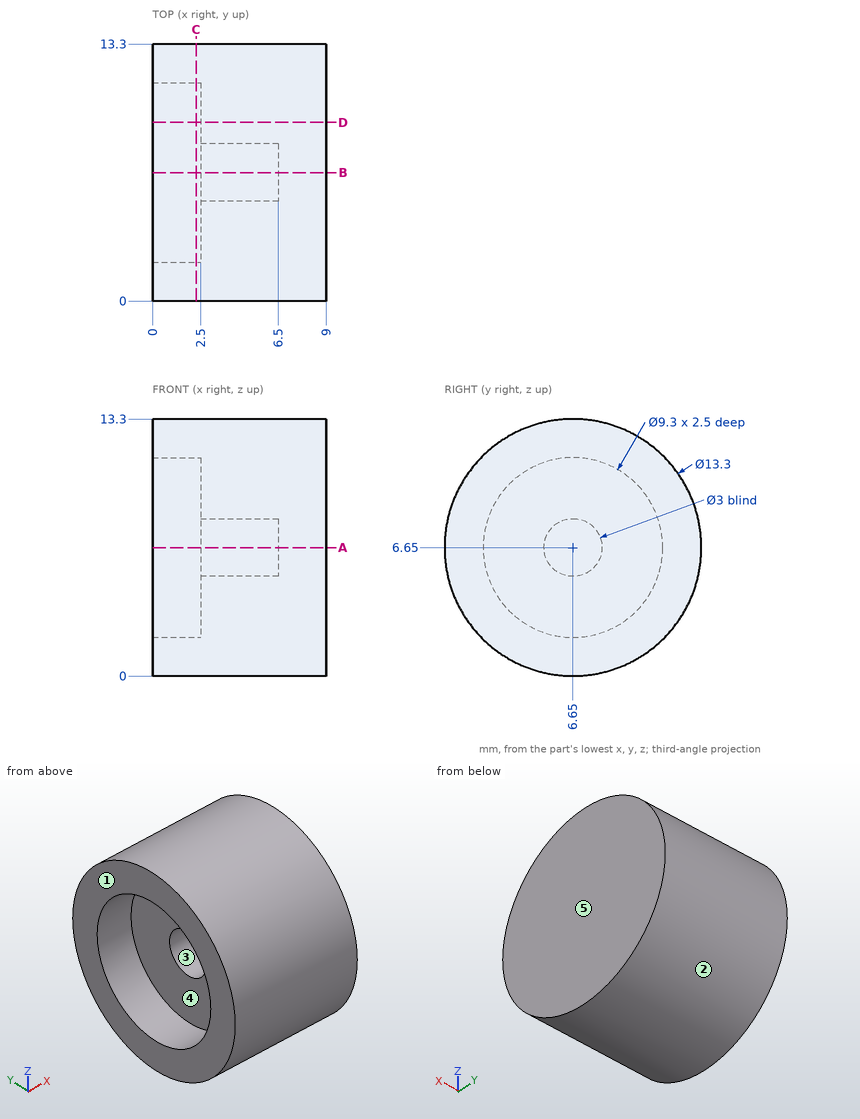
Geometry: see drawing. Coordinates: mm, zero at the bounding-box minimum. A direction names the side the tool comes from. Round coordinates to 2 decimals unless told otherwise and drop trailing zeros. Write each loop counter-clockwise with the first axis right and the second up, starting at its lowest first coordinate (ties: lowest second). Pieces come first, ordered by that corner, then holes.
1) Reachability of the marked faces 4 and 5 from +Z, -Z, +X, -X, +Y, -Y: full face, straight path, thin tool, end or side. Return the list, or none.
2) Draft query along Y for the marked faces 1, 2 and 3. Return one class per face: pulls with the +Y half, pulls with the -Y half, needs draft (parallel to the pull), parting line crosses it, or undercut.
3) Cut plane A-A (z = 6.65). Return the cut outline in (x, y).
4) Contact query for flat-ended pins moving along their axis: P1, Ø1, axis at x = 5.5, z = 9, coming from the -Y side; P2, Ø1.5, axis at y = 7, z = 7, coming from the -X side; P3, Ø2, axis at x = 2.5, y = 9, coming from the -Z side. Output: stop coordinate, or through.
5) Ray query, L1, parallel to Z at x = 1.35, y = 6.65; L2, parallel to X at y = 6, z = 4.5; L3, parallel to Z at x = 2, y = 2.75. Return the intervals inside material, ascending.
6) Cut plane C-C (x = 2.25). Return the cut outline in (y, z), then the cut area to 3 significant figures.
7) Cut plane D-D (y = 9.25). Return the cut outline in (x, z).
Geometry says:
1. face 4: -X
1. face 5: +Z, -Z, +X, +Y, -Y
2. face 1: needs draft
2. face 2: parting line crosses it
2. face 3: undercut
3. outline: (0, 0) - (9, 0) - (9, 13.3) - (0, 13.3) - (0, 11.3) - (2.5, 11.3) - (2.5, 8.15) - (6.5, 8.15) - (6.5, 5.15) - (2.5, 5.15) - (2.5, 2) - (0, 2) - close
4. P1: stops at y = 0.26
4. P2: stops at x = 6.5
4. P3: stops at z = 0.14
5. L1: z = 0 to 2, 11.3 to 13.3
5. L2: x = 2.5 to 9
5. L3: z = 1.26 to 4.12, 9.18 to 12.04
6. outline: circle Ø13.3 at (6.65, 6.65); hole circle Ø9.3 at (6.65, 6.65)
6. area: 71.0 mm2
7. outline: (0, 0.53) - (9, 0.53) - (9, 12.77) - (0, 12.77) - (0, 10.51) - (2.5, 10.51) - (2.5, 2.79) - (0, 2.79) - close
